Could you check a few things on this model? Use its own coordinates, in mm. Give positions to 0.01 mm unless a question says otherwise; leave off trailing zeros. Write each loop counter-clockwise with the first axis right and the second up, starting at its lowest first coordinate (ties: lowest second). Pieces come first, ordered by that corner, then holes. Notation, with made-up numbers: (39, 59) - (68, 59) arc R21 cw to (68, 91) - close; hole circle Ø7 at (81, -17.75). An arc over 180 degrees is marked (long way). Answer as a JSON object with one key per item and string values. Group by question number.
```python
from build123d import *

# Parameters (mm, degrees)
SALIENTE_EXTRUIR1_DEPTH = 282


with BuildPart() as part:
    # Croquis1 → Saliente-Extruir1 (new body)
    with BuildSketch(Plane.XY):
        Polygon((7.372056275, -5.675), (10, -5.675), (10, 0.5), (6, 0.5), (6, 3), (4, 3), (4, 0), (4.4, 0), (4.95, 0), (5.657106781, 0), (7.957106781, -2.3), (4.9, -2.3), (4.9, -3.202943725), align=None)
        Polygon((10, -5.675), (12.627943725, -5.675), (15.1, -3.202943725), (15.1, -2.3), (12.042893219, -2.3), (14.342893219, 0), (16, 0), (16, 3), (14, 3), (14, 0.5), (10, 0.5), align=None)
    extrude(amount=SALIENTE_EXTRUIR1_DEPTH)


solid = part.part
```
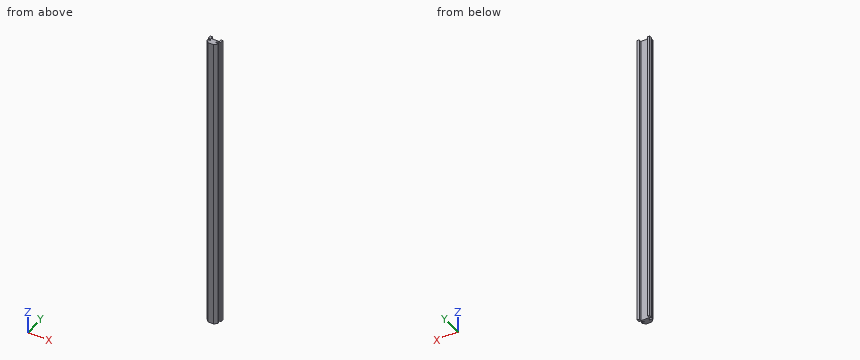
(1) Will these pins go through, and if not, where does the flat tip stop? P1, Ø2, axis at x = 6, z = 252.5, coming from the -Y side; P2, Ø0.8, axis at x = 5, z = 77.5, coming from the -Y side; P3, Ø1, axis at y = -3, z = 184.5, coming from the -X side.
(2) I need wall thicknesses on L1, parallel to X at y = 2.75, z = 64; L2, parallel to X at y = -3.25, z = 209; L3, parallel to Y at x = 15.5, z = 253.5. Which ranges of each line are inside material? Lowest first, please.
(3) I want a section at A-A, the plane z = 41. Please give me the cut outline in (x, y) (3 decimals), and give its area (3 significant figures).
Entries:
{
 "1": {"P1": "y = -5.3", "P2": "y = -3.7", "P3": "x = 4.9"},
 "2": {"L1": "4 to 6, 14 to 16", "L2": "4.95 to 15.05", "L3": "0 to 3"},
 "3": {"outline": "(4, 0) - (5.657, 0) - (7.957, -2.3) - (4.9, -2.3) - (4.9, -3.203) - (7.372, -5.675) - (12.628, -5.675) - (15.1, -3.203) - (15.1, -2.3) - (12.043, -2.3) - (14.343, 0) - (16, 0) - (16, 3) - (14, 3) - (14, 0.5) - (6, 0.5) - (6, 3) - (4, 3) - close", "area": "59.0 mm^2"}
}
